from build123d import *

# Parameters (mm, degrees)
F3_D = 18


with BuildPart() as f1:
    # F0 (on Front) → F1 (revolve)
    with BuildSketch(Plane.XZ):
        with BuildLine():
            Line((0, 584.2), (0, 0))
            Line((0, 0), (50.8, 0))
            Line((50.8, 0), (50.8, 406.4))
            ThreePointArc((50.8, 406.4), (58.2394877579, 424.3605122421), (76.2, 431.8))
            Line((76.2, 431.8), (1618.646797334, 431.8))
            Line((1618.646797334, 431.8), (2320.7796175957, 431.8))
            Line((2320.7796175957, 431.8), (2320.7796175957, 533.4))
            Line((2320.7796175957, 533.4), (2295.3796175957, 558.8))
            Line((2295.3796175957, 558.8), (1790.0687900748, 558.8))
            Line((1790.0687900748, 558.8), (1790.0687900748, 533.4))
            Line((1790.0687900748, 533.4), (1716.2160762749, 533.4))
            Line((1716.2160762749, 533.4), (1716.2160762749, 635))
            Line((1716.2160762749, 635), (50.8, 635))
            ThreePointArc((50.8, 635), (14.8789755157, 620.1210244843), (0, 584.2))
        make_face()
    revolve(axis=Axis((25.4, 0, 0), (-1, 0, 0)))

    # F3 (through all)
    with Locations(Plane(origin=(0, 0, 0), x_dir=(0, -1, 0), z_dir=(-1, 0, 0))):
        with Locations((0, 0)):
            Hole(F3_D / 2)


solid = f1.part
The model under review builds one solid part; all positions refer to its coordinate system, in mm. A direction names the side the tool comes from. Round coordinates to 2 decimals unless told otherwise and drop trailing zeros. Loops run counter-clockwise (first coordinate to the right, second up) from the corner with the lowest first, then second, coordinate; pieces in that order, holes last. Notation, with made-up numbers: M 34,84.5 L 91,84.5 A22 cw 91,106.5 Z; hole C -34.5,10.5 d7. An arc over 180 degrees is marked long. Answer as a JSON object with one key per item and string values.
Item 1: Clearance check with flat-ended pins moving along their axes: P1, Ø8, axis at y = -461.5, z = 405.5, coming from the -X side; P2, Ø3, axis at x = 1506.5, y = -501.5, coming from the +Z side; P3, Ø1.5, axis at x = 1187, z = 76.5, coming from the -Y side. State where each tip first meets the part, or that it passes through.
Check sheet entries:
{"P1": "x = 7.24", "P2": "z = 391.44", "P3": "y = -630.47"}
Item 2: The part is to be moulded in two halves that separate along X. For faces 4 (the face through (2320.78, 2, -432)), 5 (the face through (1752.63, 160.22, 508.77)), 6 (the face through (2039.187, -340.021, -443.445)), 7 (the face through (0, 8, -8)), say which applies: +X half, -X half, draft (parallel to the pull), parting line (faces both ways), or undercut.
Check sheet entries:
{"face 4": "+X half", "face 5": "undercut", "face 6": "draft", "face 7": "-X half"}
Item 3: We need section A-A, the plane x = 2105. State the section outline as (y, z) points, and give its area (3 significant figures).
Check sheet entries:
{"outline": "C 0,0 d1117.6; hole C 0,0 d863.6", "area": "395,000 mm2"}
Item 4: Tool access review of faces 1 (the face through (50.8, 6, -85)), 2 (the face through (1716.216, 520, 144)), 3 (the face through (871.85, 190.737, 605.677)): name each direction out of +Z, -Z, +X, -X, +Y, -Y from which nothing blocks a thin tool from reaching the whole face with its end or side.
Check sheet entries:
{"face 1": "+X", "face 2": "none", "face 3": "+X, -X"}
Item 5: We need section B-B, the plane x = 1684.5. State the section outline as (y, z) points.
Check sheet entries:
{"outline": "C 0,0 d1270; hole C 0,0 d863.6"}
Item 6: For line 1 along Z through (x, y) = (1469, -1); line 2 along Z through (x, y) = (1304.5, 7); line 3 along X through (y, z) = (-204, -53), list the stretches that pass through material, from the lowest coordinate up.
Check sheet entries:
{"line 1": "-635 to -431.8, 431.8 to 635", "line 2": "-634.96 to -431.74, 431.74 to 634.96", "line 3": "0 to 50.8"}
